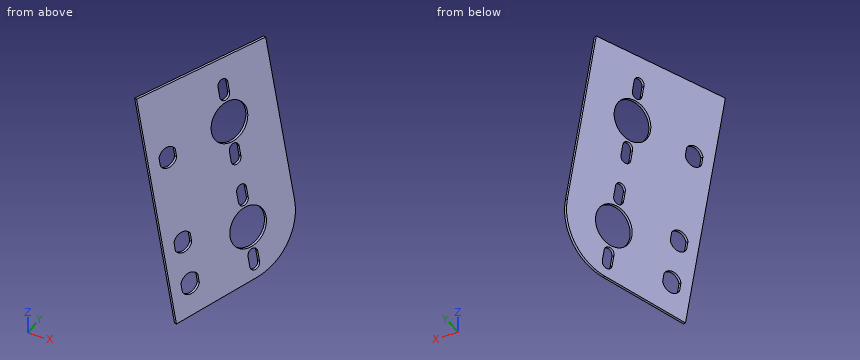
from build123d import *

# Parameters (mm, degrees)
SKETCH39_R          = 12.065
BOSS_EXTRUDE1_DEPTH = 1.5875


with BuildPart() as part:
    # Sketch39 → Boss-Extrude1 (new body)
    with BuildSketch(Plane(origin=(-441.521969452, 172.104793819, -62.182961286), x_dir=(-0.1212218165913434, 0.04725213510134498, 0.9915001295565519), z_dir=(-0.9237984742451071, 0.36009566214142513, -0.1301056996804562))):
        with BuildLine():
            Line((-228.748442373, 213.554448141), (-90.363815922, 201.963804234))
            Line((-90.363815922, 201.963804234), (-90.363815922, 287.351743879))
            Line((-90.363815922, 287.351743879), (-190.640017459, 295.750550698))
            ThreePointArc((-190.640017459, 295.750550698), (-213.325518758, 288.505331466), (-224.243446911, 267.341116014))
            Line((-224.243446911, 267.341116014), (-228.748442373, 213.554448141))
        make_face()
        with Locations(Location((-128.463815922, 259.318927244, 0), (0, 0, 270))):
            Circle(SKETCH39_R, mode=Mode.SUBTRACT)
        with Locations(Location((-193.237014843, 264.74411863, 0), (0, 0, 270))):
            Circle(SKETCH39_R, mode=Mode.SUBTRACT)
        with BuildLine():
            Line((-211.461957069, 230.522345777), (-206.270039744, 230.087487755))
            ThreePointArc((-206.270039744, 230.087487755), (-203.136411518, 224.15373677), (-207.213438794, 218.823926718))
            Line((-207.213438794, 218.823926718), (-212.405356118, 219.25878474))
            ThreePointArc((-212.405356118, 219.25878474), (-215.538984345, 225.192535724), (-211.461957069, 230.522345777))
        make_face(mode=Mode.SUBTRACT)
        with BuildLine():
            Line((-186.168382291, 228.189847508), (-180.976464967, 227.754989487))
            ThreePointArc((-180.976464967, 227.754989487), (-178.017364976, 222.049847551), (-181.884267338, 216.916429257))
            Line((-181.884267338, 216.916429257), (-187.076184662, 217.351287279))
            ThreePointArc((-187.076184662, 217.351287279), (-190.035284653, 223.056429214), (-186.168382291, 228.189847508))
        make_face(mode=Mode.SUBTRACT)
        with BuildLine():
            Line((-215.859429659, 269.914226569), (-209.53158638, 269.384227103))
            ThreePointArc((-209.53158638, 269.384227103), (-206.55149466, 265.859295931), (-210.076425831, 262.879204212))
            Line((-210.076425831, 262.879204212), (-216.40426911, 263.409203678))
            ThreePointArc((-216.40426911, 263.409203678), (-219.38436083, 266.934134849), (-215.859429659, 269.914226569))
        make_face(mode=Mode.SUBTRACT)
        with BuildLine():
            Line((-170.614600027, 259.57401069), (-176.942443306, 260.104010157))
            ThreePointArc((-176.942443306, 260.104010157), (-179.922535026, 263.628941328), (-176.397603855, 266.609033048))
            Line((-176.397603855, 266.609033048), (-170.069760576, 266.079033581))
            ThreePointArc((-170.069760576, 266.079033581), (-167.089668856, 262.55410241), (-170.614600027, 259.57401069))
        make_face(mode=Mode.SUBTRACT)
        with BuildLine():
            Line((-151.086230738, 264.489035183), (-144.758387459, 263.959035717))
            ThreePointArc((-144.758387459, 263.959035717), (-141.778295739, 260.434104546), (-145.30322691, 257.454012826))
            Line((-145.30322691, 257.454012826), (-151.631070189, 257.984012292))
            ThreePointArc((-151.631070189, 257.984012292), (-154.611161909, 261.508943463), (-151.086230738, 264.489035183))
        make_face(mode=Mode.SUBTRACT)
        with BuildLine():
            Line((-105.841401106, 254.148819304), (-112.169244385, 254.678818771))
            ThreePointArc((-112.169244385, 254.678818771), (-115.149336105, 258.203749942), (-111.624404934, 261.183841662))
            Line((-111.624404934, 261.183841662), (-105.296561655, 260.653842195))
            ThreePointArc((-105.296561655, 260.653842195), (-102.316469935, 257.128911024), (-105.841401106, 254.148819304))
        make_face(mode=Mode.SUBTRACT)
        with BuildLine():
            Line((-134.050869929, 223.824655055), (-128.858952604, 223.389797033))
            ThreePointArc((-128.858952604, 223.389797033), (-125.899852614, 217.684655097), (-129.766754976, 212.551236803))
            Line((-129.766754976, 212.551236803), (-134.9586723, 212.986094825))
            ThreePointArc((-134.9586723, 212.986094825), (-137.917772291, 218.691236761), (-134.050869929, 223.824655055))
        make_face(mode=Mode.SUBTRACT)
    extrude(amount=BOSS_EXTRUDE1_DEPTH)


solid = part.part
Geometry check sheet. Reference: the model listing, model coordinates, mm. Round coordinates to 2 decimals unless told otherwise and drop trailing zeros. Write each loop counter-clockwise with the first axis right and the second up, starting at its lowest first coordinate (ties: lowest second). Pieces come first, ordered by that corner, then holes. Notation, with made-up numbers: (-2, -3) -> (33, -3) arc R31 cw to (33, 25) -> close; hole circle Ø4 at (-13, 19). An arc over 180 degrees is marked (long way). One line per item, written item: value. Start each with the question number.
(1) Cross-section at C-C, the plane x = -355. Record the cut outline in (y, z), and give its area (3 significant figures).
(2) Cross-section at A-A, the plane y = 372.5. Give the number of separate pieces and of enclosed holes in the cut face, and give its area (3 significant figures).
(3) Go/stop test with flat-tipped pins: pin 1 Ø5 at (y, z) = (366.5, -255.5) entering from -X; pin 2 Ø6 at (y, z) = (420, -226.5) entering from -X; pin 3 Ø1 at (y, z) = (382, -267) entering from +X. Record where each tip stops, or that it passes through.
(4) Cross-section at B-B, the plane y = 394.5. Record the cut outline in (x, z).
(5) Scan lines: line 1 (X direction, y = 432, z = -240); line 2 (X direction, y = 420.5, z = -183). Record each from-to range of solid material in increasing order. Write a range as [from, to].
Answer:
1. outline: (356.46, -166.28) -> (357.33, -176.08) -> (366.03, -151.99) -> (361.7, -151.78) -> close
1. area: 85.1 mm²
2. separate pieces: 4
2. enclosed holes: 0
2. area: 176 mm²
3. pin 1: x = -341.28
3. pin 2: x = -324.71
3. pin 3: x = -330.65
4. outline: (-343.9, -151.99) -> (-325, -286.21) -> (-323.32, -285.95) -> (-342.21, -151.78) -> close
5. line 1: [-316.89, -315.17]
5. line 2: [-329.4, -327.68]
